Part model, mm, in its own coordinate system. Face numbers are marked on the shaded views. A direction names the side the tool comes from. Coordinates: 2 decimals unless noted, no trailing zeros. Order: outer loops, then holes, each group sorted by start corner. A loop starts at its lowest first (then second) coordinate and runs counter-clockwise, first axis right, second up. Notation, with made-up numbers: (-26, -38.75) - (16, -38.75) arc R22 ccw to (16, -2.75) - close; hole circle Ø4 at (19, -32). An arc over 180 degrees is marked (long way). Use a Markdown table: item, result. Add a question column.
1) Saw through at C-C on z = 6. Count the separate pieces of the cut face and the enclosed holes in it, then the cut area to 3 significant figures.
2) Tool access for the marked faces 3, 4 and 5: list every direction of +Z, -Z, +X, -X, +Y, -Y with a clear straight run to the whole face (end or side of a thin tool).
3) Drop flat-ended pins along their axis: P1, Ø4, axis at x = -4, y = -12, coming from the +Z side; P2, Ø1.1, axis at x = 4.5, y = 28.5, coming from the +Z side. Give the stop position or say it passes through.
4) Saw through at D-D on x = -2. List the corners of the cut face in (y, z), then the cut area to 3 significant figures.
5) Wall check: L1, parallel to X at y = -2, z = 1.75; L2, parallel to Y at x = -14.5, z = 1.5; L3, parallel to X at y = 22, z = 1. Give the ranges that are in metal, low to high. Write a range as [from, to].
6) Saw through at B-B on y = 0. List the corners of the cut face in (x, z).
7) Saw through at A-A on x = 15. List the corners of the cut face in (y, z).
8) Two-plate mould, pull along X, no slides. Class the marked faces 1 and 2: +X half, -X half, draft (parallel to the pull), parting line (faces both ways), or undercut.
```python
from build123d import *

# Parameters (mm, degrees)
F0_W      = 35.814
F0_H      = 51.054
F1_DEPTH  = 7.9375
F2_W      = 5.588
F2_H      = 17.68475
F2_H_2    = 10.4775
F3_DEPTH  = 25.4
F5_DEPTH  = 1.27
F6_W      = 18.288
F6_H      = 44.323
F7_DEPTH  = 5.08
F8_W      = 18.288
F8_H      = 4.1275
F9_DEPTH  = 25.4
F10_W     = 18.288
F10_H     = 1.016
F11_DEPTH = 3.175


with BuildPart() as f1:
    # F0 (on Top) → F1 (new body)
    with BuildSketch(Plane.XY):
        with Locations((0.853188, 7.523157)):
            Rectangle(F0_W, F0_H)
    extrude(amount=F1_DEPTH)

    # F2 (on face) → F3 (cut)
    with BuildSketch(Plane.XY.offset(7.9375)):
        with Locations((-12.672312, 22.620282)):
            Rectangle(F2_W, F2_H)
        with Locations((-12.672312, 7.523157)):
            Rectangle(F2_W, F2_H_2)
        with Locations((-12.672312, -7.573968)):
            Rectangle(F2_W, F2_H)
        with Locations((14.378688, -7.573968)):
            Rectangle(F2_W, F2_H)
        with Locations((14.378688, 7.523157)):
            Rectangle(F2_W, F2_H_2)
        with Locations((14.378688, 22.620282)):
            Rectangle(F2_W, F2_H)
    extrude(amount=-F3_DEPTH, mode=Mode.SUBTRACT)

    # F4 (on face) → F5 (cut)
    with BuildSketch(Plane.XY.offset(7.9375)):
        Polygon((11.584688, 28.922657), (-9.878312, 28.922657), (-9.878312, 13.777907), (-9.878312, 12.761907), (-9.878312, 2.284407), (-9.878312, 1.268407), (-9.878312, -16.416343), (11.584688, -16.416343), (11.584688, 1.268407), (11.584688, 2.284407), (11.584688, 12.761907), (11.584688, 13.777907), align=None)
    extrude(amount=-F5_DEPTH, mode=Mode.SUBTRACT)

    # F6 (on face) → F7 (cut)
    with BuildSketch(Plane.XY.offset(6.6675)):
        with Locations((0.853188, 5.745157)):
            Rectangle(F6_W, F6_H)
    extrude(amount=-F7_DEPTH, mode=Mode.SUBTRACT)

    # F8 (on face) → F9 (cut)
    with BuildSketch(Plane.XY.offset(7.9375)):
        with Locations((0.853188, 30.986407)):
            Rectangle(F8_W, F8_H)
    extrude(amount=-F9_DEPTH, mode=Mode.SUBTRACT)

    # F10 (on face) → F11 (cut)
    with BuildSketch(Plane.XY.offset(6.6675)):
        with Locations((0.853188, 28.414657)):
            Rectangle(F10_W, F10_H)
    extrude(amount=-F11_DEPTH, mode=Mode.SUBTRACT)


solid = f1.part
```
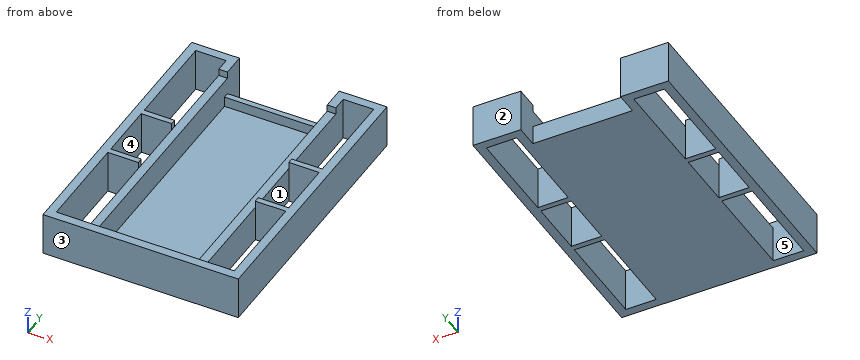
Results are:
| question | item | result |
|---|---|---|
| 1 | separate pieces | 1 |
| 1 | enclosed holes | 6 |
| 1 | area | 411 mm2 |
| 2 | face 3 | +Z, -Z, +X, -X, -Y |
| 2 | face 4 | +Z, -Z |
| 2 | face 5 | +Z |
| 3 | P1 | z = 1.59 |
| 3 | P2 | z = 3.49 |
| 4 | outline | (-18, 0) - (28.92, 0) - (28.92, 3.49) - (27.91, 3.49) - (27.91, 1.59) - (-16.42, 1.59) - (-16.42, 7.94) - (-18, 7.94) - close |
| 4 | area | 86.5 mm2 |
| 5 | L1 | [-17.05, -15.47], [-9.88, -8.29], [10, 11.58], [17.17, 18.76] |
| 5 | L2 | [-18, -16.42], [1.27, 2.28], [12.76, 13.78], [31.46, 33.05] |
| 5 | L3 | [-17.05, -15.47], [-9.88, 11.58], [17.17, 18.76] |
| 6 | outline | (-17.05, 0) - (-15.47, 0) - (-15.47, 7.94) - (-17.05, 7.94) - close; (-9.88, 0) - (11.58, 0) - (11.58, 6.67) - (10, 6.67) - (10, 1.59) - (-8.29, 1.59) - (-8.29, 6.67) - (-9.88, 6.67) - close; (17.17, 0) - (18.76, 0) - (18.76, 7.94) - (17.17, 7.94) - close |
| 7 | outline | (-18, 0) - (-16.42, 0) - (-16.42, 7.94) - (-18, 7.94) - close; (1.27, 0) - (2.28, 0) - (2.28, 7.94) - (1.27, 7.94) - close; (12.76, 0) - (13.78, 0) - (13.78, 7.94) - (12.76, 7.94) - close; (31.46, 0) - (33.05, 0) - (33.05, 7.94) - (31.46, 7.94) - close |
| 8 | face 1 | undercut |
| 8 | face 2 | draft |
